Build history of the part. All positions in model axes, mm. Coordinates: 2 decimals unless noted, no trailing zeros. Order: outer loops, then holes, each group sorted by start corner. A loop starts at its lowest first (then second) coordinate and runs counter-clockwise, first axis right, second up. Notation, with made-up numbers: M 6,51 L 53,51 A30 ccw 53,76 Z; hole C -30,77.25 d1. An arc over 180 degrees is marked long. Write item = value, one per line. Start each with the question number.
Q1. Drill centre lines: probe 1 along X at (y, z) = (22.75, -82); probe 2 along Z at (x, y) = (120, 22). Where is each one in solid material? Low to high.
Q2. Pin check, flat tips, straight feed: P1, Ø7, axis at x = 3.5, y = 23.5, coming from the +Z side; P2, Ø2, axis at x = 125, z = -12.5, coming from the +Y side; P3, Ø4, axis at y = 15.875, z = -115.275, coming from the -X side. Stop position of each tip, or through.
Q3. Band-saw the part on A-A on z = -239. Write the cut outline in (x, y).
Q4. Band-saw the part on B-B on x = 30.5. Write the cut outline in (y, z) (3 decimals).
```python
from build123d import *

# Parameters (mm, degrees)
SKETCH1_W           = 427.3
SKETCH1_H           = 319.3
BOSS_EXTRUDE1_DEPTH = 25.4
CUT_EXTRUDE1_DEPTH  = 19.05
SKETCH6_W           = 427.3
SKETCH6_H           = 6.5
CUT_EXTRUDE4_DEPTH  = 6.35
SKETCH4_R           = 3.175
CUT_EXTRUDE2_DEPTH  = 38.1
CUT_EXTRUDE3_START  = -38.1
SKETCH5_R           = 3.175
CUT_EXTRUDE3_DEPTH  = 38.1


with BuildPart() as part:
    # Sketch1 → Boss-Extrude1 (new body)
    with BuildSketch(Plane(origin=(0, 0, 0), x_dir=(1, 0, 0), z_dir=(0, 1, 0))):
        with Locations((213.65, 159.65)):
            Rectangle(SKETCH1_W, SKETCH1_H)
    extrude(amount=BOSS_EXTRUDE1_DEPTH)

    # Sketch2 → Cut-Extrude1 (cut)
    with BuildSketch(Plane(origin=(0, 25.4, 0), x_dir=(1, 0, 0), z_dir=(0, 1, 0))):
        Polygon((410.8, 302.8), (410.8, 16.5), (410.8, 10), (410.8, 0), (417.3, 0), (417.3, 10), (417.3, 16.5), (417.3, 302.8), (417.3, 309.3), (417.3, 319.3), (410.8, 319.3), (410.8, 309.3), align=None)
        Polygon((16.5, 16.5), (16.5, 302.8), (16.5, 309.3), (16.5, 319.3), (10, 319.3), (10, 309.3), (10, 302.8), (10, 16.5), (10, 10), (10, 0), (16.5, 0), (16.5, 10), align=None)
    extrude(amount=-CUT_EXTRUDE1_DEPTH, mode=Mode.SUBTRACT)

    # Sketch6 → Cut-Extrude4 (cut)
    with BuildSketch(Plane(origin=(0, 25.4, 0), x_dir=(1, 0, 0), z_dir=(0, 1, 0))):
        with Locations((213.65, 13.25)):
            Rectangle(SKETCH6_W, SKETCH6_H)
        with Locations((213.65, 306.05)):
            Rectangle(SKETCH6_W, SKETCH6_H)
    extrude(amount=-CUT_EXTRUDE4_DEPTH, mode=Mode.SUBTRACT)

    # Sketch4 → Cut-Extrude2 (cut)
    with BuildSketch(Plane(origin=(427.3, 0, 0), x_dir=(0, 0, -1), z_dir=(1, 0, 0))):
        with Locations((115.275, 15.875)):
            Circle(SKETCH4_R)
        with Locations((230.775, 15.875)):
            Circle(SKETCH4_R)
    extrude(amount=-CUT_EXTRUDE2_DEPTH, mode=Mode.SUBTRACT)

    # Sketch5 → Cut-Extrude3 (cut)
    with BuildSketch(Plane.ZY.offset(CUT_EXTRUDE3_START)):
        with Locations(Location((-230.775, 15.875, 0), (0, 0, 180))):
            Circle(SKETCH5_R)
        with Locations(Location((-115.275, 15.875, 0), (0, 0, 180))):
            Circle(SKETCH5_R)
    extrude(amount=CUT_EXTRUDE3_DEPTH, mode=Mode.SUBTRACT)


solid = part.part
```
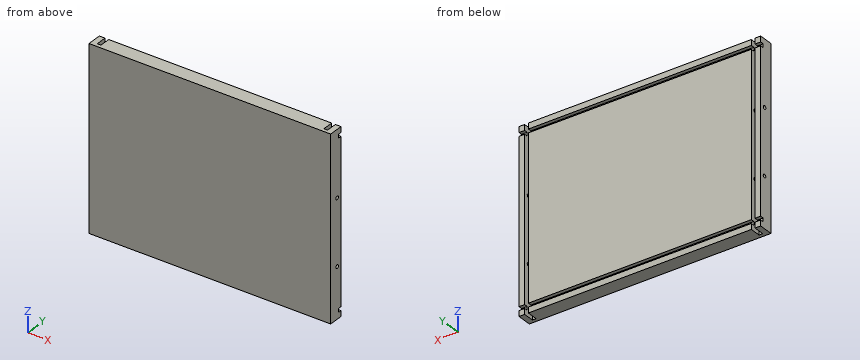
Recorded:
q1.probe_1 = 0 to 10, 16.5 to 410.8, 417.3 to 427.3
q1.probe_2 = -319.3 to -309.3, -302.8 to -16.5, -10 to 0
q2.P1 = 0
q2.P2 = 19.05
q2.P3 = 38.1
q3.outline = M 0,0 L 427.3,0 L 427.3,25.4 L 417.3,25.4 L 417.3,6.35 L 410.8,6.35 L 410.8,25.4 L 16.5,25.4 L 16.5,6.35 L 10,6.35 L 10,25.4 L 0,25.4 Z
q4.outline = M 0,-319.3 L 25.4,-319.3 L 25.4,-309.3 L 19.05,-309.3 L 19.05,-302.8 L 25.4,-302.8 L 25.4,-16.5 L 19.05,-16.5 L 19.05,-10 L 25.4,-10 L 25.4,0 L 0,0 Z; hole C 15.875,-230.775 d6.35; hole C 15.875,-115.275 d6.35
